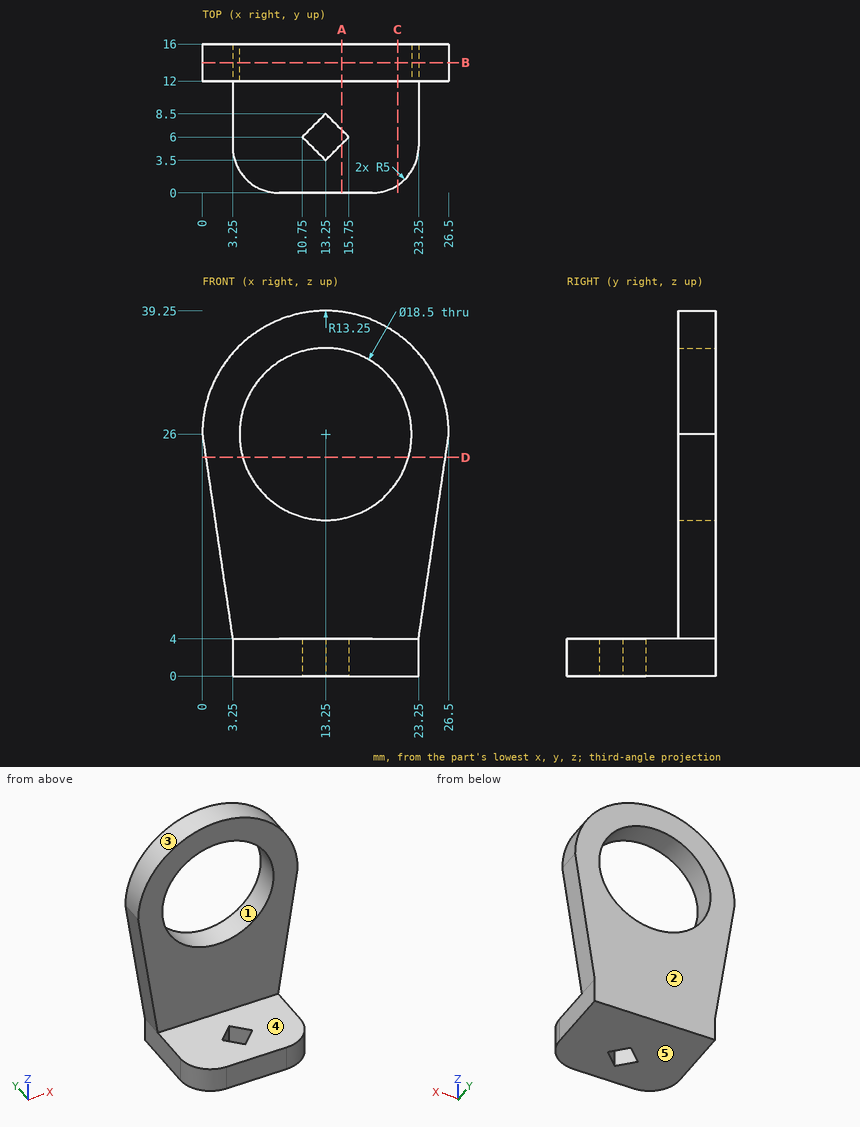
Design review of the part shown in the three views and the two pictorial views. Dimensions are in mm from the part's minimum x, y and z. A direction names the side the tool comes from. Round coordinates to 2 decimals unless told otherwise and drop trailing zeros. Write each loop counter-clockwise with the first axis right and the second up, starting at its lowest first coordinate (ties: lowest second). Pieces come first, ordered by that corner, then holes. Notation, with made-up numbers: (5, -16) - (26, -16) arc R29 ccw to (26, 4) - close; hole circle Ø4 at (-16.5, -32.5). An arc over 180 degrees is marked (long way). Answer as CSV lines item,"result". Start each with the question number.
(1) Add section A-A, the plane x = 15. State the section outline as (y, z) points.
(2) Add section B-B, the plane y = 14. State the section outline as (x, z) points, plus the area to 3 significant figures.
(3) Add section D-D, the plane z = 23.5. State the section outline as (x, y) points, plus the area to 3 significant figures.
(4) Add section C-C, the plane x = 21. State the section outline as (y, z) points, plus the area to 3 significant figures.
(5) Mouldability with a two-part tool opening along Z and no side actions: class the marked faces 1, 2 and 3 as +Z half, -Z half, draft (parallel to the pull), parting line (faces both ways), or undercut.
(6) Machinability: for the marked faces 4 and 5, which of the approach directions +Z, -Z, +X, -X, +Y, -Y give a long, thin tool a straight path to every point of the face, cutting with its end or side? Answer none if there is none.
(7) For pin 1 (6 mm diameter, centred on x = 11.5, z = 14.5, fed in from -Y); pin 2 (1.5 mm diameter, centred on y = 10.5, z = 35, fed in from -X); pin 3 (4.5 mm diameter, centred on y = 11.5, z = 1.5, fed in from +X); pin 4 (4.5 mm diameter, centred on y = 9, z = 2.5, fed in from -X), all flat-tipped, find the tip position at first contact; note any pin that passes through.
(8) For line 1 (Z direction, x = 13.25, y = 13.15); line 2 (Y direction, x = 22.25, z = 13.5); line 3 (Z direction, x = 4.5, y = 6.5), list the stretches that pass through material, from the lowest coordinate up.
From the geometry:
1,outline,"(0, 0) - (5.25, 0) - (5.25, 4) - (0, 4) - close; (6.75, 0) - (16, 0) - (16, 16.92) - (12, 16.92) - (12, 4) - (6.75, 4) - close; (12, 35.08) - (16, 35.08) - (16, 39.13) - (12, 39.13) - close"
2,outline,"(0, 26) - (3.25, 4) - (3.25, 0) - (23.25, 0) - (23.25, 4) - (26.5, 26) arc R13.25 ccw to start; hole circle Ø18.5 at (13.25, 26)"
2,area,"598 mm²"
3,outline,"(0.37, 12) - (4.34, 12) - (4.34, 16) - (0.37, 16) - close; (22.16, 12) - (26.13, 12) - (26.13, 16) - (22.16, 16) - close"
3,area,"31.8 mm²"
4,outline,"(0.82, 0) - (16, 0) - (16, 20.95) - (12, 20.95) - (12, 4) - (0.82, 4) - close; (12, 31.05) - (16, 31.05) - (16, 36.75) - (12, 36.75) - close"
4,area,"151 mm²"
5,face 1,"undercut"
5,face 2,"draft"
5,face 3,"+Z half"
6,face 4,"+Z, +X, -X, -Y"
6,face 5,"-Z, +X, -X, +Y, -Y"
7,pin 1,"stops at y = 12"
7,pin 2,"passes through"
7,pin 3,"stops at x = 23.25"
7,pin 4,"stops at x = 3.25"
8,line 1,"z = 0 to 16.75, 35.25 to 39.25"
8,line 2,"y = 12 to 16"
8,line 3,"z = 0 to 4"
